Check sheet for the modelled part. Datum: model origin and axes. Units: mm. A direction names the side the tool comes from. Give positions to 0.01 mm unless a question says otherwise; leave off trailing zeros. Write each loop counter-clockwise with the first axis right and the second up, starting at its lowest first coordinate (ties: lowest second). Pieces come first, ordered by that corner, then holes. Notation, with made-up numbers: (2.25, 84) -> (61.25, 84) arc R12 ccw to (61.25, 100) -> close; hole circle Ø6 at (83.5, 18). An arc over 180 degrees is marked (long way). Answer as a JSON object with one key per item and string values.
from build123d import *

# Parameters (mm, degrees)
BOSS_EXTRUDE1_DEPTH = 1.5
SKETCH2_R           = 10
BOSS_EXTRUDE2_DEPTH = 10
SKETCH3_R           = 2.5
CUT_EXTRUDE1_DEPTH  = 2.5
CUT_EXTRUDE2_DEPTH  = 4
CUT_EXTRUDE3_DEPTH  = 2
CUT_EXTRUDE4_DEPTH  = 2


with BuildPart() as part:
    # Sketch1 → Boss-Extrude1 (new body)
    with BuildSketch(Plane(origin=(0, 0, 0), x_dir=(1, 0, 0), z_dir=(0, 1, 0))):
        with BuildLine():
            add(Edge.make_bspline(
                [(7.183697139, 7.183697139), (0, 87.002554241), (-7.183697139, 7.183697139)],
                knots=[1.862253121, 1.862253121, 1.862253121, 4.420932186, 4.420932186, 4.420932186], degree=2, weights=[1, 0.287347886, 1]))
            add(Edge.make_bspline(
                [(-7.183697139, 7.183697139), (-87.002554241, 0), (-7.183697139, -7.183697139)],
                knots=[5.003845775, 5.003845775, 5.003845775, 7.562524839, 7.562524839, 7.562524839], degree=2, weights=[1, 0.287347886, 1]))
            add(Edge.make_bspline(
                [(-7.183697139, -7.183697139), (0, -87.002554241), (7.183697139, -7.183697139)],
                knots=[5.003845775, 5.003845775, 5.003845775, 7.562524839, 7.562524839, 7.562524839], degree=2, weights=[1, 0.287347886, 1]))
            add(Edge.make_bspline(
                [(7.183697139, -7.183697139), (87.002554241, 0), (7.183697139, 7.183697139)],
                knots=[1.862253121, 1.862253121, 1.862253121, 4.420932186, 4.420932186, 4.420932186], degree=2, weights=[1, 0.287347886, 1]))
        make_face()
    extrude(amount=BOSS_EXTRUDE1_DEPTH)

    # Sketch2 → Boss-Extrude2 (add)
    with BuildSketch(Plane(origin=(0, 1.5, 0), x_dir=(1, 0, 0), z_dir=(0, 1, 0))):
        Circle(SKETCH2_R)
    extrude(amount=BOSS_EXTRUDE2_DEPTH)

    # Sketch3 → Cut-Extrude1 (cut)
    with BuildSketch(Plane.XZ):
        Circle(SKETCH3_R)
    extrude(amount=-CUT_EXTRUDE1_DEPTH, mode=Mode.SUBTRACT)

    # Sketch4 → Cut-Extrude2 (cut)
    with BuildSketch(Plane(origin=(0, 11.5, 0), x_dir=(1, 0, 0), z_dir=(0, 1, 0))):
        with BuildLine():
            add(Edge.make_bspline(
                [(-2.354354779, -2.354354779), (0, -20.812496246), (2.354354779, -2.354354779)],
                knots=[5.055412921, 5.055412921, 5.055412921, 7.510957694, 7.510957694, 7.510957694], degree=2, weights=[1, 0.336336397, 1]))
            add(Edge.make_bspline(
                [(2.354354779, -2.354354779), (20.812496246, 0), (2.354354779, 2.354354779)],
                knots=[1.913820267, 1.913820267, 1.913820267, 4.36936504, 4.36936504, 4.36936504], degree=2, weights=[1, 0.336336397, 1]))
            add(Edge.make_bspline(
                [(2.354354779, 2.354354779), (0, 20.812496246), (-2.354354779, 2.354354779)],
                knots=[1.913820267, 1.913820267, 1.913820267, 4.36936504, 4.36936504, 4.36936504], degree=2, weights=[1, 0.336336397, 1]))
            add(Edge.make_bspline(
                [(-2.354354779, 2.354354779), (-20.812496246, 0), (-2.354354779, -2.354354779)],
                knots=[5.055412921, 5.055412921, 5.055412921, 7.510957694, 7.510957694, 7.510957694], degree=2, weights=[1, 0.336336397, 1]))
        make_face()
    extrude(amount=-CUT_EXTRUDE2_DEPTH, mode=Mode.SUBTRACT)

    # Sketch5 → Cut-Extrude3 (cut)
    with BuildSketch(Plane(origin=(0, 7.5, 0), x_dir=(1, 0, 0), z_dir=(0, 1, 0))):
        with BuildLine():
            ThreePointArc((7, 0), (6.467156728, 2.678784027), (4.949747468, 4.949747468))
            add(Edge.make_bspline(
                [(4.949747468, 4.949747468), (4.13981345, 5.759681487), (1.89338429, 4.571034031)],
                knots=[3.141592654, 3.141592654, 3.141592654, 4.000843717, 4.000843717, 4.000843717], degree=2, weights=[1, 0.909121791, 1]))
            add(Edge.make_bspline(
                [(1.89338429, 4.571034031), (1.145419674, 7), (0, 7)],
                knots=[2.282341591, 2.282341591, 2.282341591, 3.141592654, 3.141592654, 3.141592654], degree=2, weights=[1, 0.909121791, 1]))
            ThreePointArc((0, 7), (-2.678784027, 6.467156728), (-4.949747468, 4.949747468))
            add(Edge.make_bspline(
                [(-4.949747468, 4.949747468), (-5.759681487, 4.13981345), (-4.571034031, 1.89338429)],
                knots=[0, 0, 0, 0.859251063, 0.859251063, 0.859251063], degree=2, weights=[1, 0.909121791, 1]))
            add(Edge.make_bspline(
                [(-4.571034031, 1.89338429), (-7, 1.145419674), (-7, 0)],
                knots=[5.423934244, 5.423934244, 5.423934244, 6.283185307, 6.283185307, 6.283185307], degree=2, weights=[1, 0.909121791, 1]))
            ThreePointArc((-7, 0), (-6.467156728, -2.678784027), (-4.949747468, -4.949747468))
            add(Edge.make_bspline(
                [(-4.949747468, -4.949747468), (-4.13981345, -5.759681487), (-1.89338429, -4.571034031)],
                knots=[0, 0, 0, 0.859251063, 0.859251063, 0.859251063], degree=2, weights=[1, 0.909121791, 1]))
            add(Edge.make_bspline(
                [(-1.89338429, -4.571034031), (-1.145419674, -7), (0, -7)],
                knots=[5.423934244, 5.423934244, 5.423934244, 6.283185307, 6.283185307, 6.283185307], degree=2, weights=[1, 0.909121791, 1]))
            ThreePointArc((0, -7), (2.678784027, -6.467156728), (4.949747468, -4.949747468))
            add(Edge.make_bspline(
                [(4.949747468, -4.949747468), (5.759681487, -4.13981345), (4.571034031, -1.89338429)],
                knots=[3.141592654, 3.141592654, 3.141592654, 4.000843717, 4.000843717, 4.000843717], degree=2, weights=[1, 0.909121791, 1]))
            add(Edge.make_bspline(
                [(4.571034031, -1.89338429), (7, -1.145419674), (7, 0)],
                knots=[2.282341591, 2.282341591, 2.282341591, 3.141592654, 3.141592654, 3.141592654], degree=2, weights=[1, 0.909121791, 1]))
        make_face()
    extrude(amount=CUT_EXTRUDE3_DEPTH, mode=Mode.SUBTRACT)

    # Sketch6 → Cut-Extrude4 (cut)
    with BuildSketch(Plane(origin=(0, 7.5, 0), x_dir=(1, 0, 0), z_dir=(0, 1, 0))):
        with BuildLine():
            add(Edge.make_bspline(
                [(-3.329560459, 0), (-14.716657229, -14.716657229), (0, -3.329560459)],
                knots=[5.055412921, 5.055412921, 5.055412921, 7.510957694, 7.510957694, 7.510957694], degree=2, weights=[1, 0.336336397, 1]))
            add(Edge.make_bspline(
                [(0, -3.329560459), (14.716657229, -14.716657229), (3.329560459, 0)],
                knots=[1.913820267, 1.913820267, 1.913820267, 4.36936504, 4.36936504, 4.36936504], degree=2, weights=[1, 0.336336397, 1]))
            add(Edge.make_bspline(
                [(3.329560459, 0), (14.716657229, 14.716657229), (0, 3.329560459)],
                knots=[1.913820267, 1.913820267, 1.913820267, 4.36936504, 4.36936504, 4.36936504], degree=2, weights=[1, 0.336336397, 1]))
            add(Edge.make_bspline(
                [(0, 3.329560459), (-14.716657229, 14.716657229), (-3.329560459, 0)],
                knots=[5.055412921, 5.055412921, 5.055412921, 7.510957694, 7.510957694, 7.510957694], degree=2, weights=[1, 0.336336397, 1]))
        make_face()
    extrude(amount=-CUT_EXTRUDE4_DEPTH, mode=Mode.SUBTRACT)


solid = part.part
1. Access from +Z, -Z, +X, -X, +Y, -Y to the whole of each face (thin tool, end or side, straight path). Record for faces 1 (the face through (-0.54, 1.23, -2.44)), 2 (the face through (6, 0, 0)), 3 (the face through (6.5, 8.5, -2.6)).
Determined:
{"face 1": "-Y", "face 2": "+Z, -Z, +X, -X, -Y", "face 3": "none"}
2. Go/stop test with flat-tipped pins: P1, Ø6, axis at x = -15, y = 9, coming from the +Z side; P2, Ø3, axis at x = -14.5, y = 1.5, coming from the -Z side. Record where each tip stops, or that it passes through.
Determined:
{"P1": "through", "P2": "z = -6.41"}
3. Sectioned sample at A-A, the plane y = 3.25. Enter the section's corners in (x, z), plus the area to 3 significant figures.
Determined:
{"outline": "circle Ø20 at (0, 0)", "area": "314 mm^2"}
4. Mould release check, pull along Y, two halves, no side actions. Record for faces 4 (the face through (-3, 11.5, 3)), 5 (the face through (-5, 7.5, 1)), 6 (the face through (-2.17, 6.43, 9.76)): released by +Y, released by -Y, zero draft, split by the parting line, or undercut.
Determined:
{"face 4": "released by +Y", "face 5": "undercut", "face 6": "zero draft"}
5. Scan lines: L1, parallel to Z at x = 0, y = 2; L2, parallel to Y at x = 3.5, z = 2.5; L3, parallel to Z at x = 0, y = 1.1. Record each from-to range of solid material in increasing order. Write a range as [from, to].
Determined:
{"L1": "[-10, -2.5], [2.5, 10]", "L2": "[0, 5.5], [9.5, 11.5]", "L3": "[-25, -2.5], [2.5, 25]"}
